The figure shows three views and two pictorial views of one solid part (mm, origin at its lowest corner). Answer the questions. A direction names the side the tool comes from. Give positions to 0.01 mm unless a question says otherwise; leave off trailing zeros. Loops run counter-clockwise (first coordinate to the right, second up) from the corner with the lowest first, then second, coordinate; pieces in that order, holes last. Notation, with made-up numbers: (21, 15.25) -> (49, 15.25) arc R25 ccw to (49, 29.25) -> close; hole circle Ø3 at (10, 60.25). An arc over 180 degrees is marked (long way). One line per item, written item: value. Start each with the question number.
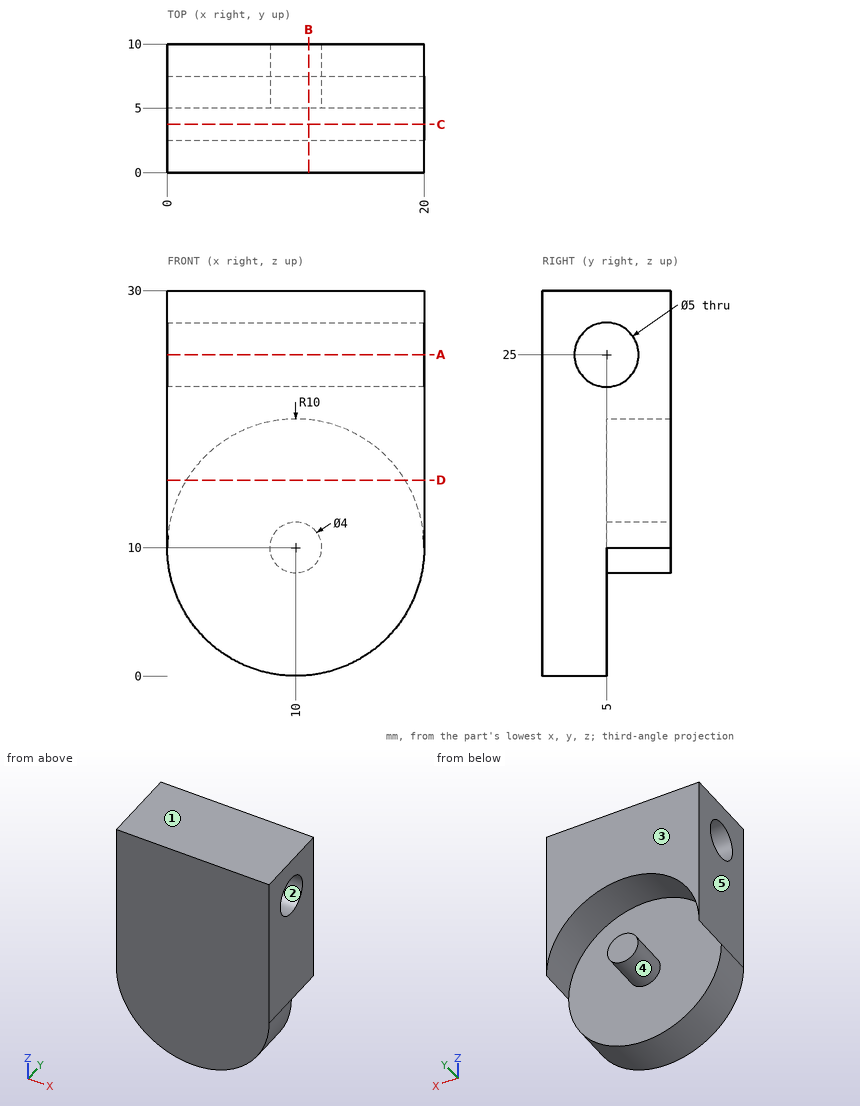
Item 1: Section A-A, the plane z = 25 is taken. Determine the outline of the cut face in (x, y), plus the area to 3 significant figures.
Item 2: Section B-B, the plane x = 11 is taken. Determine the outline of the cut face in (y, z).
Item 3: For the marked faces 4 and 5, determine the directions among +Z, -Z, +X, -X, +Y, -Y from which every point of the face is accessible in a straight line to the end or side of a thin tool.
Item 4: Section C-C, the plane y = 3.75 is taken. Determine the outline of the cut face in (x, z).
Item 5: Determine the mould class of the marked faces 1, 2 and 3 for opening direction Z: pulls with the +Z half, pulls with the -Z half, needs draft (parallel to the pull), parting line crosses it, or undercut.
Item 6: Consider L1, parallel to Y at x = 8.5, z = 25; L2, parallel to Y at x = 4, z = 17.75; L3, parallel to Z at x = 7.25, y = 3. Determine where each line is inside the solid, lowest interval first. Write a range as [from, to].
Item 7: Section D-D, the plane z = 15.25 is taken. Determine the outline of the cut face in (x, y).
Computed values:
1. outline: (0, 0) -> (20, 0) -> (20, 2.5) -> (0, 2.5) -> close; (0, 7.5) -> (20, 7.5) -> (20, 10) -> (0, 10) -> close
1. area: 100 mm²
2. outline: (0, 0.05) -> (5, 0.05) -> (5, 8.27) -> (10, 8.27) -> (10, 11.73) -> (5, 11.73) -> (5, 19.95) -> (10, 19.95) -> (10, 30) -> (0, 30) -> close; hole circle Ø5 at (5, 25)
3. face 4: +Y
3. face 5: +Z, -Z, -X, +Y, -Y
4. outline: (0, 10) arc R10 ccw to (20, 10) -> (20, 22.83) -> (0, 22.83) -> close; (0, 27.17) -> (20, 27.17) -> (20, 30) -> (0, 30) -> close
5. face 1: pulls with the +Z half
5. face 2: undercut
5. face 3: needs draft
6. L1: [0, 2.5], [7.5, 10]
6. L2: [0, 5]
6. L3: [0.39, 23.5], [26.5, 30]
7. outline: (0, 0) -> (20, 0) -> (20, 10) -> (18.51, 10) -> (18.51, 5) -> (1.49, 5) -> (1.49, 10) -> (0, 10) -> close
